Geometry: final body of the model. Coordinates: model frame, mm. Face numbers are marked on the shaded views. A direction names the side the tool comes from. Give positions to 0.01 mm unless a question says otherwise; leave off trailing zeros. Write each loop counter-clockwise with the first axis right and the second up, starting at its lowest first coordinate (ties: lowest second). Pieces come first, ordered by that corner, then holes.
Q1. Mould query, pull axis X, two halves, no side actions, for the marked faces 1, 2, 3 and 4. Classes: +X half, -X half, draft (parallel to the pull), parting line (faces both ways), or undercut.
Q2. Section B-B (z = 7). Return the cut outline in (x, y).
Q3. Section A-A (y = 12.5). Return the cut outline in (x, z).
Q4. Reachability of the marked faces 5 and 6 from +Z, -Z, +X, -X, +Y, -Y: full face, straight path, thin tool, end or side. Return the list, or none.
Q5. Pin query (flat end, axial travel): pin 1 Ø5 at (x, y) = (51, 16) entering from +Z; pin 2 Ø1.5 at (y, z) = (15, 4.5) entering from -X; pin 3 Ø2 at (y, z) = (21, 6.5) entering from -X. Return the tip coordinate at first contact, or that it passes through.
Q6. Section D-D (x = -4.5). Return the cut outline in (y, z), plus the area to 3 significant figures.
Q7. Line query: line 1 (Y direction, x = 50, z = 6.6); line 2 (X direction, y = 14.75, z = 6.5); line 3 (X direction, y = 13, z = 1.75). Output: solid intervals per line, ascending.
Q8. Section C-C (z = 1). Return the cut outline in (x, y), plus the area to 3 significant figures.
from build123d import *

# Parameters (mm, degrees)
SKETCH1_R           = 12.5
SKETCH1_W           = 50
SKETCH1_H           = 25
BOSS_EXTRUDE2_DEPTH = 5
CUT_EXTRUDE3_REACH  = 69.5
SKETCH3_R           = 3.5
SKETCH3_3_R         = 9.5
SKETCH3_3_R_2       = 8
BOSS_EXTRUDE3_DEPTH = 3


with BuildPart() as part:
    # Sketch1 → Boss-Extrude2 (new body)
    with BuildSketch(Plane.XY):
        with Locations((0, 12.5)):
            Circle(SKETCH1_R)
        with Locations((50, 12.5)):
            Circle(SKETCH1_R)
        with Locations((25, 12.5)):
            Rectangle(SKETCH1_W, SKETCH1_H)
    extrude(amount=BOSS_EXTRUDE2_DEPTH)

    # Sketch3 → Cut-Extrude3 (cut, up to next)
    with BuildSketch(Plane.XY.offset(5), mode=Mode.PRIVATE) as cut_extrude3_sk1:
        with Locations((0, 12.5)):
            Circle(SKETCH3_R)
    cut_extrude3_tool1 = extrude(cut_extrude3_sk1.sketch, amount=-CUT_EXTRUDE3_REACH, mode=Mode.PRIVATE) & part.part
    # Sketch3 → Cut-Extrude3 (cut, up to next)
    with BuildSketch(Plane.XY.offset(5), mode=Mode.PRIVATE) as cut_extrude3_sk2:
        with Locations((50, 12.5)):
            Circle(SKETCH3_R)
    cut_extrude3_tool2 = extrude(cut_extrude3_sk2.sketch, amount=-CUT_EXTRUDE3_REACH, mode=Mode.PRIVATE) & part.part
    add(cut_extrude3_tool1.solids().sort_by_distance((0, 12.5, 5))[0], mode=Mode.SUBTRACT)
    add(cut_extrude3_tool2.solids().sort_by_distance((50, 12.5, 5))[0], mode=Mode.SUBTRACT)

    # Sketch3<3> → Boss-Extrude3 (add)
    # profile 1 of 2: a face of its own
    with BuildSketch(Plane.XY.offset(5)):
        with Locations((0, 12.5)):
            Circle(SKETCH3_3_R)
        with Locations((0, 12.5)):
            Circle(SKETCH3_3_R_2, mode=Mode.SUBTRACT)
    # profile 2 of 2: a face of its own
    with BuildSketch(Plane.XY.offset(5)):
        with Locations((50, 12.5)):
            Circle(SKETCH3_3_R)
        with Locations((50, 12.5)):
            Circle(SKETCH3_3_R_2, mode=Mode.SUBTRACT)
    extrude(amount=BOSS_EXTRUDE3_DEPTH)


solid = part.part
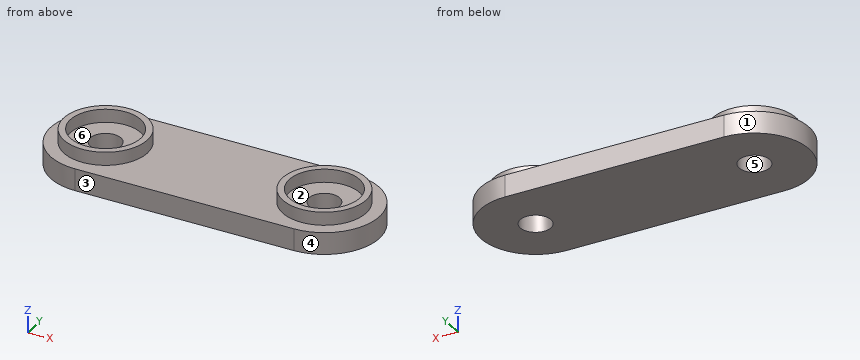
Computed:
1. face 1: -X half
1. face 2: undercut
1. face 3: draft
1. face 4: +X half
2. outline: circle Ø19 at (0, 12.5); circle Ø19 at (50, 12.5); hole circle Ø16 at (0, 12.5); hole circle Ø16 at (50, 12.5)
3. outline: (-12.5, 0) - (-3.5, 0) - (-3.5, 5) - (-8, 5) - (-8, 8) - (-9.5, 8) - (-9.5, 5) - (-12.5, 5) - close; (3.5, 0) - (46.5, 0) - (46.5, 5) - (42, 5) - (42, 8) - (40.5, 8) - (40.5, 5) - (9.5, 5) - (9.5, 8) - (8, 8) - (8, 5) - (3.5, 5) - close; (53.5, 0) - (62.5, 0) - (62.5, 5) - (59.5, 5) - (59.5, 8) - (58, 8) - (58, 5) - (53.5, 5) - close
4. face 5: +Z, -Z
4. face 6: +Z
5. pin 1: stops at z = 5
5. pin 2: stops at x = -12.38
5. pin 3: stops at x = -5.83
6. outline: (0.84, 0) - (24.16, 0) - (24.16, 5) - (20.87, 5) - (20.87, 8) - (19.11, 8) - (19.11, 5) - (5.89, 5) - (5.89, 8) - (4.13, 8) - (4.13, 5) - (0.84, 5) - close
6. area: 127 mm2
7. line 1: y = 3 to 4.5, 20.5 to 22
7. line 2: x = -9.23 to -7.68, 7.68 to 9.23, 40.77 to 42.32, 57.68 to 59.23
7. line 3: x = -12.49 to -3.46, 3.46 to 46.54, 53.46 to 62.49
8. outline: (0, 0) - (50, 0) arc R12.5 ccw to (50, 25) - (0, 25) arc R12.5 ccw to start; hole circle Ø7 at (0, 12.5); hole circle Ø7 at (50, 12.5)
8. area: 1,660 mm2
